Source: three-view drawing plus pictorial views. Frame: mm from the lowest corner of the part. A direction names the side the tool comes from. Round coordinates to 2 decimals unless told otherwise and drop trailing zeros. Order: outer loops, then holes, each group sorted by start corner. A loop starts at its lowest first (then second) coordinate and runs counter-clockwise, first axis right, second up. Notation, with made-up numbers: (53, 66) -> (112, 66) arc R22 cw to (112, 91) -> close; hole circle Ø6 at (17.5, 77). An arc over 180 degrees is marked (long way). Answer as CSV lines item,"result".
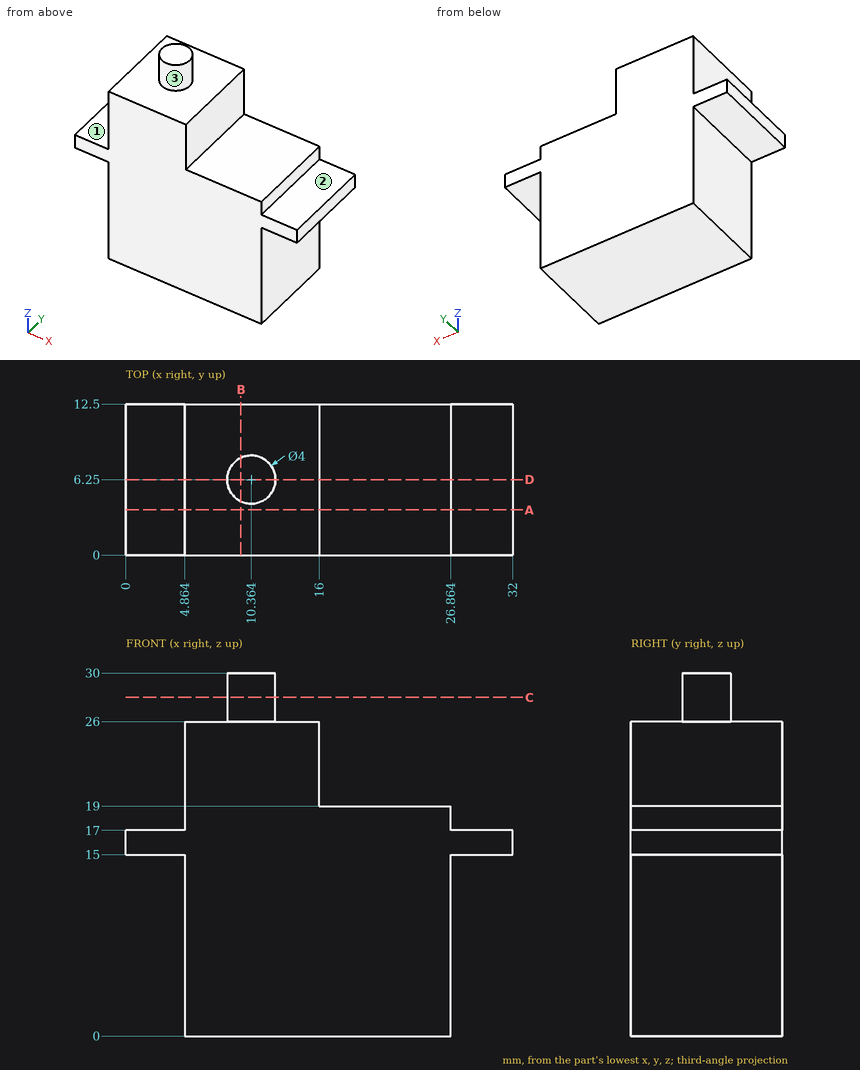
1. Line query: L1, parallel to X at y = 2, z = 7.5; L2, parallel to Z at x = 3, y = 8.5; L3, parallel to X at y = 2.5, z = 20.25. Output: solid intervals per line, ascending. Write a range as [from, to].
Results below:
L1,"[4.86, 26.86]"
L2,"[15, 17]"
L3,"[4.86, 16]"
2. Section query C-C on z = 28. Return loops of the section in (x, y).
Results below:
outline,"circle Ø4 at (10.36, 6.25)"
3. Section query B-B on x = 9.5. Return loops of the section in (y, z), and give its area (3 significant figures).
Results below:
outline,"(0, 0) -> (12.5, 0) -> (12.5, 26) -> (8.05, 26) -> (8.05, 30) -> (4.45, 30) -> (4.45, 26) -> (0, 26) -> close"
area,"339 mm2"
4. Reachability of the marked faces 1, 2 and 3 from +Z, -Z, +X, -X, +Y, -Y: full face, straight path, thin tool, end or side. Return the list, or none.
Results below:
face 1,"+Z, -X, +Y, -Y"
face 2,"+Z, +X, +Y, -Y"
face 3,"+Z"
5. Section query A-A on y = 3.75. Return loops of the section in (x, z).
Results below:
outline,"(0, 15) -> (4.86, 15) -> (4.86, 0) -> (26.86, 0) -> (26.86, 15) -> (32, 15) -> (32, 17) -> (26.86, 17) -> (26.86, 19) -> (16, 19) -> (16, 26) -> (4.86, 26) -> (4.86, 17) -> (0, 17) -> close"
6. Section query D-D on y = 6.25. Return loops of the section in (x, z), and give its area (3 significant figures).
Results below:
outline,"(0, 15) -> (4.86, 15) -> (4.86, 0) -> (26.86, 0) -> (26.86, 15) -> (32, 15) -> (32, 17) -> (26.86, 17) -> (26.86, 19) -> (16, 19) -> (16, 26) -> (12.36, 26) -> (12.36, 30) -> (8.36, 30) -> (8.36, 26) -> (4.86, 26) -> (4.86, 17) -> (0, 17) -> close"
area,"532 mm2"
7. Pin query (flat end, axial travel): pin 1 (2.5 mm diameter, centred on x = 30, y = 5.5, fed in from +Z); pin 2 (1 mm diameter, centred on y = 5, z = 18.5, fed in from +X); pin 3 (3.5 mm diameter, centred on y = 4, z = 24, fed in from +X). Return the tip coordinate at first contact, or that it passes through.
Results below:
pin 1,"z = 17"
pin 2,"x = 26.86"
pin 3,"x = 16"
